Model file for the job. Use its own axes, mm. Face numbers are marked on the shaded views. A direction names the side the tool comes from. Give positions to 0.01 mm unless a question says otherwise; leave off trailing zeros. Write each loop counter-clockwise with the first axis right and the second up, starting at its lowest first coordinate (ties: lowest second). Pieces come first, ordered by that corner, then holes.
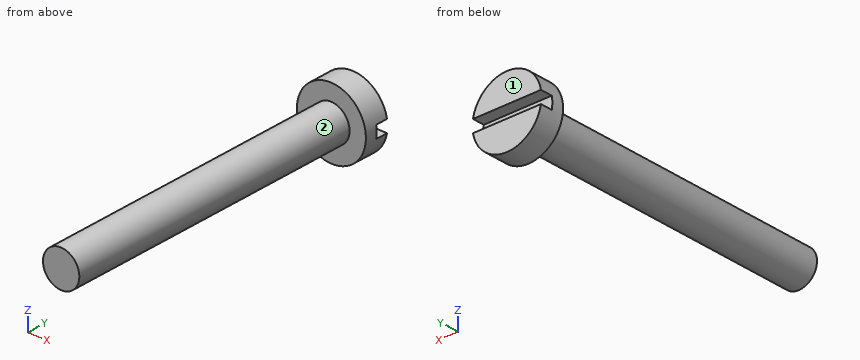
```python
from build123d import *

# Parameters (mm, degrees)
SKETCH1_R           = 2.85
BOSS_EXTRUDE1_DEPTH = 2
SKETCH2_R           = 1.5
BOSS_EXTRUDE2_DEPTH = 25
SKETCH3_W           = 6
SKETCH3_H           = 1
CUT_EXTRUDE1_DEPTH  = 1


with BuildPart() as part:
    # Sketch1 → Boss-Extrude1 (new body)
    with BuildSketch(Plane(origin=(0, 0, 0), x_dir=(1, 0, 0), z_dir=(0, 1, 0))):
        with Locations(Location((0, 0, 0), (0, 0, 270))):
            Circle(SKETCH1_R)
    extrude(amount=BOSS_EXTRUDE1_DEPTH)

    # Sketch2 → Boss-Extrude2 (add)
    with BuildSketch(Plane(origin=(0, 0, 0), x_dir=(1, 0, 0), z_dir=(0, 1, 0))):
        with Locations(Location((0, 0, 0), (0, 0, 270))):
            Circle(SKETCH2_R)
    extrude(amount=-BOSS_EXTRUDE2_DEPTH)

    # Sketch3 → Cut-Extrude1 (cut)
    with BuildSketch(Plane(origin=(0, 2, 0), x_dir=(1, 0, 0), z_dir=(0, 1, 0))):
        Rectangle(SKETCH3_W, SKETCH3_H)
    extrude(amount=-CUT_EXTRUDE1_DEPTH, mode=Mode.SUBTRACT)


solid = part.part
```
1. Pin check, flat tips, straight feed: P1, Ø1, axis at x = 1.5, y = -11.5, coming from the +Z side; P2, Ø0.5, axis at x = 0.5, y = 1.5, coming from the +Z side. Stop position of each tip, or through.
Calculated:
P1: stops at z = 1.12
P2: stops at z = 2.84
2. Slice it at C-C, the plane y = -12.25. Write the cut outline in (x, z).
Calculated:
outline: circle Ø3 at (0, 0)
3. Slice it at D-D, the plane z = 1. Write the cut outline in (x, y), and give its area (3 significant figures).
Calculated:
outline: (-2.67, 0) - (-1.12, 0) - (-1.12, -25) - (1.12, -25) - (1.12, 0) - (2.67, 0) - (2.67, 2) - (-2.67, 2) - close
area: 66.6 mm2
4. Slice it at A-A, the plane x = 0. Write the cut outline in (y, z), and give its area (3 significant figures).
Calculated:
outline: (-25, -1.5) - (0, -1.5) - (0, -2.85) - (2, -2.85) - (2, -0.5) - (1, -0.5) - (1, 0.5) - (2, 0.5) - (2, 2.85) - (0, 2.85) - (0, 1.5) - (-25, 1.5) - close
area: 85.4 mm2
5. Slice it at B-B, the plane z = 0. Write the cut outline in (x, y), and give its area (3 significant figures).
Calculated:
outline: (-2.85, 0) - (-1.5, 0) - (-1.5, -25) - (1.5, -25) - (1.5, 0) - (2.85, 0) - (2.85, 1) - (-2.85, 1) - close
area: 80.7 mm2
6. Probe probe 1 along Y at (x, z) = (2.4, -0.8); probe 2 along Y at (x, z) = (-0.45, 0.1); probe 3 along Z at (x, y) = (-0.2, -7). List the from-to ranges inside material, lowest first.
Calculated:
probe 1: y = 0 to 2
probe 2: y = -25 to 1
probe 3: z = -1.49 to 1.49
7. Which spindle directions (+Z, -Z, +X, -X, +Y, -Y) get a long thin tool onto all of the face, cutting with end or side? Do the marked faces 1 and 2. Say none if no direction does.
Calculated:
face 1: +Z, -Z, +X, -X, +Y
face 2: -Y
